```python
from build123d import *

# Parameters (mm, degrees)
BOSS_EXTRUDE1_DEPTH = 9
BOSS_EXTRUDE2_DEPTH = 8
BOSS_EXTRUDE3_DEPTH = 8
BOSS_EXTRUDE4_DEPTH = 8


with BuildPart() as part:
    # Sketch2 → Boss-Extrude1 (new, symmetric)
    with BuildSketch(Plane.XY):
        with BuildLine():
            ThreePointArc((-25.130575003, -25.130575003), (-35.54, 0), (-25.130575003, 25.130575003))
            Line((-25.130575003, 25.130575003), (-25.837681785, 25.837681785))
            ThreePointArc((-25.837681785, 25.837681785), (-36.54, 0), (-25.837681785, -25.837681785))
            Line((-25.837681785, -25.837681785), (-25.130575003, -25.130575003))
        make_face()
    extrude(amount=BOSS_EXTRUDE1_DEPTH, both=True)

    # Sketch3 → Boss-Extrude2 (add, symmetric)
    with BuildSketch(Plane.XY):
        with BuildLine():
            ThreePointArc((-25.837681785, 25.837681785), (-33.599252383, 16.491716629), (-37.54, 5))
            Line((-37.54, 5), (-37.54, 0))
            Line((-37.54, 0), (-37.54, -5))
            ThreePointArc((-37.54, -5), (-33.599252383, -16.491716629), (-25.837681785, -25.837681785))
            ThreePointArc((-25.837681785, -25.837681785), (-36.54, 0), (-25.837681785, 25.837681785))
        make_face()
    extrude(amount=BOSS_EXTRUDE2_DEPTH, both=True)



with BuildPart() as body_2:
    # Sketch4 → Boss-Extrude3 (new, symmetric)
    with BuildSketch(Plane.XY):
        with BuildLine():
            Line((-42.54, 5), (-42.54, -5))
            ThreePointArc((-42.54, -5), (-36.829168158, -17.535179295), (-25.837681785, -25.837681785))
            ThreePointArc((-25.837681785, -25.837681785), (-51.675363569, 0), (-25.837681785, 25.837681785))
            ThreePointArc((-25.837681785, 25.837681785), (-36.829168158, 17.535179295), (-42.54, 5))
        make_face()
    extrude(amount=BOSS_EXTRUDE3_DEPTH, both=True)


with BuildPart() as part_1:
    add(part.part)

    add(body_2.part)  # Boss-Extrude4 merges body 2
    # Sketch5 → Boss-Extrude4 (add, symmetric)
    with BuildSketch(Plane.XY):
        with BuildLine():
            Line((-42.54, 5), (-37.54, 5))
            ThreePointArc((-37.54, 5), (-33.599252383, 16.491716629), (-25.837681785, 25.837681785))
            ThreePointArc((-25.837681785, 25.837681785), (-36.829168158, 17.535179295), (-42.54, 5))
        make_face()
        with BuildLine():
            Line((-42.54, -5), (-37.54, -5))
            ThreePointArc((-37.54, -5), (-33.599252383, -16.491716629), (-25.837681785, -25.837681785))
            ThreePointArc((-25.837681785, -25.837681785), (-36.829168158, -17.535179295), (-42.54, -5))
        make_face()
    extrude(amount=BOSS_EXTRUDE4_DEPTH, both=True)


solid = part_1.part
```
Model file for the job. Use its own axes, mm. A direction names the side the tool comes from. Give positions to 0.01 mm unless a question says otherwise; leave off trailing zeros. Write each loop counter-clockwise with the first axis right and the second up, starting at its lowest first coordinate (ties: lowest second). Pieces come first, ordered by that corner, then holes. Notation, with made-up numbers: (36, 73) -> (40, 73) arc R14 ccw to (40, 98) -> close; hole circle Ø4 at (-1, 54). An arc over 180 degrees is marked (long way). Use CSV: the item, a comma, the result in double quotes. Start each with the question number.
1) Cut at B-B on z = 4. List the corners of the cut face in (x, y).
2) Cut at C-C on x = -30.5. List the corners of the cut face in (y, z), plus the area to 3 significant figures.
3) Drill centre lines: L1, parallel to Z at x = -47.75, y = 8; L2, parallel to X at y = -4, z = -3.5; L3, parallel to Y at x = -26.25, z = -7.5. Where is each one in solid material? Low to high.
4) Pin check, flat tips, straight feed: P1, Ø2, axis at y = 14.5, z = 2, coming from the -X side; P2, Ø3, axis at y = 0.5, z = 2, coming from the +X side; P3, Ø4, axis at y = -6, z = -2.5, coming from the +X side; P4, Ø3, axis at x = -34.5, y = 12.5, coming from the +Z side. Stop position of each tip, or through.
5) Two-plate mould, pull along Y, no slides. Class faces 1 (the flat face through (-37.54, 0, 0)), 2 (the flat face through (-36, 2, 9)), 3 (the cylindrical face through (-36.538, 0.402, -8.493)): released by +Y, released by -Y, zero draft, split by the parting line, or undercut.
6) Tool access for faces 4 (the flat face through (-44, 0, -8)), 5 (the cylindrical face through (-36.538, 0.402, 8.507)), 6 (the flat face through (-40, 5, 0)): list every direction of +Z, -Z, +X, -X, +Y, -Y with a clear straight run to the whole face (end or side of a thin tool).
7) Cut at A-A on y = 0. List the corners of the cut face in (x, z).
8) Cut at D-D on y = -19.5. List the corners of the cut face in (x, z), plus the area to 3 significant figures.
Final values:
1,outline,"(-25.84, -25.84) -> (-25.13, -25.13) arc R35.54 cw to (-25.13, 25.13) -> (-25.84, 25.84) arc R25.84 ccw to start; hole (-42.54, -5) -> (-37.54, -5) -> (-37.54, 5) -> (-42.54, 5) -> close"
2,outline,"(-25.41, -8) -> (-20.12, -8) -> (-20.12, -9) -> (-18.24, -9) -> (-18.24, 9) -> (-20.12, 9) -> (-20.12, 8) -> (-25.41, 8) -> close; (18.24, -9) -> (20.12, -9) -> (20.12, -8) -> (25.41, -8) -> (25.41, 8) -> (20.12, 8) -> (20.12, 9) -> (18.24, 9) -> close"
2,area,"237 mm2"
3,L1,"z = -8 to 8"
3,L2,"x = -51.36 to -42.54, -37.54 to -35.31"
3,L3,"y = -25.83 to -23.96, 23.96 to 25.83"
4,P1,"stops at x = -47.87"
4,P2,"stops at x = -35.48"
4,P3,"stops at x = -34.63"
4,P4,"stops at z = 9"
5,face 1,"undercut"
5,face 2,"zero draft"
5,face 3,"split by the parting line"
6,face 4,"-Z, -X"
6,face 5,"+Z, -X"
6,face 6,"+Z, -Z"
7,outline,"(-51.68, -8) -> (-42.54, -8) -> (-42.54, 8) -> (-51.68, 8) -> close; (-37.54, -8) -> (-36.54, -8) -> (-36.54, -9) -> (-35.54, -9) -> (-35.54, 9) -> (-36.54, 9) -> (-36.54, 8) -> (-37.54, 8) -> close"
8,outline,"(-42.79, -8) -> (-30.9, -8) -> (-30.9, -9) -> (-29.71, -9) -> (-29.71, 9) -> (-30.9, 9) -> (-30.9, 8) -> (-42.79, 8) -> close"
8,area,"212 mm2"
